from build123d import *

# Parameters (mm, degrees)
F1_DEPTH = 50.8
F3_DEPTH = 40.64
F0_R     = 12.7
F4_DEPTH = 50.8
F5_DEPTH = 38.1


with BuildPart() as f1:
    # F0 (on Front) → F1 (new body)
    with BuildSketch(Plane.XZ):
        with BuildLine():
            Line((-63.5, -50.8), (63.5, -50.8))
            ThreePointArc((63.5, -50.8), (72.480256, -47.080256), (76.2, -38.1))
            Line((76.2, -38.1), (76.2, 38.1))
            ThreePointArc((76.2, 38.1), (72.480256, 47.080256), (63.5, 50.8))
            Line((63.5, 50.8), (-63.5, 50.8))
            ThreePointArc((-63.5, 50.8), (-72.480256, 47.080256), (-76.2, 38.1))
            Line((-76.2, 38.1), (-76.2, -38.1))
            ThreePointArc((-76.2, -38.1), (-72.480256, -47.080256), (-63.5, -50.8))
        make_face()
    extrude(amount=-F1_DEPTH)

    # F2 (on face) → F3 (cut)
    with BuildSketch(Plane.XZ):
        with BuildLine():
            Line((-57.15, -44.45), (57.15, -44.45))
            ThreePointArc((57.15, -44.45), (66.130256, -40.730256), (69.85, -31.75))
            Line((69.85, -31.75), (69.85, 31.75))
            ThreePointArc((69.85, 31.75), (66.130256, 40.730256), (57.15, 44.45))
            Line((57.15, 44.45), (-57.15, 44.45))
            ThreePointArc((-57.15, 44.45), (-66.130256, 40.730256), (-69.85, 31.75))
            Line((-69.85, 31.75), (-69.85, -31.75))
            ThreePointArc((-69.85, -31.75), (-66.130256, -40.730256), (-57.15, -44.45))
        make_face()
    extrude(amount=-F3_DEPTH, mode=Mode.SUBTRACT)

    # F0 (on Front) → F4 (join)
    with BuildSketch(Plane.XZ):
        Polygon((-63.5, 50.8), (63.5, 50.8), (63.5, 76.2), (63.5, 101.6), (0, 101.6), (-38.1, 101.6), (-63.5, 101.6), align=None)
        with BuildLine():
            ThreePointArc((-25.4, 76.2), (-47.080256, 67.219744), (-38.1, 88.9))
            ThreePointArc((-38.1, 88.9), (-29.119744, 85.180256), (-25.4, 76.2))
        make_face(mode=Mode.SUBTRACT)
        with BuildLine():
            ThreePointArc((21.59, 76.2), (-15.266435, 60.933565), (0, 97.79))
            ThreePointArc((0, 97.79), (15.266435, 91.466435), (21.59, 76.2))
        make_face(mode=Mode.SUBTRACT)
        with Locations((38.1, 76.2)):
            Circle(F0_R, mode=Mode.SUBTRACT)
        with Locations((38.1, 76.2)):
            Circle(F0_R)
        with BuildLine():
            ThreePointArc((21.59, 76.2), (15.266435, 91.466435), (0, 97.79))
            ThreePointArc((0, 97.79), (-15.266435, 60.933565), (21.59, 76.2))
        make_face()
        with BuildLine():
            ThreePointArc((-25.4, 76.2), (-29.119744, 85.180256), (-38.1, 88.9))
            ThreePointArc((-38.1, 88.9), (-47.080256, 67.219744), (-25.4, 76.2))
        make_face()
    extrude(amount=-F4_DEPTH)

    # F0 (on Front) → F5 (cut)
    with BuildSketch(Plane.XZ):
        with BuildLine():
            ThreePointArc((-25.4, 76.2), (-29.119744, 85.180256), (-38.1, 88.9))
            ThreePointArc((-38.1, 88.9), (-47.080256, 67.219744), (-25.4, 76.2))
        make_face()
        with BuildLine():
            ThreePointArc((21.59, 76.2), (15.266435, 91.466435), (0, 97.79))
            ThreePointArc((0, 97.79), (-15.266435, 60.933565), (21.59, 76.2))
        make_face()
        with Locations((38.1, 76.2)):
            Circle(F0_R)
    extrude(amount=-F5_DEPTH, mode=Mode.SUBTRACT)


solid = f1.part
Input: part model. Units: mm. Frame: model coordinates. A direction names the side the tool comes from. Round coordinates to 2 decimals unless told otherwise and drop trailing zeros. Order: outer loops, then holes, each group sorted by start corner. A loop starts at its lowest first (then second) coordinate and runs counter-clockwise, first axis right, second up.
1. Set-up query: faces 4 (the face through (38, 38.1, 76)), 5 (the face through (-63.5, 25, 77)), 6 (the face through (1, 25, 101.6)). Return all of +Z, -Z, +X, -X, +Y, -Y with unobstructed straight access to the full face (end or side cutting, diameter ignored); none if empty.
The answers:
face 4: -Y
face 5: +Z, -X, +Y, -Y
face 6: +Z, +X, -X, +Y, -Y
2. Mould query, pull axis X, two halves, no side actions, for faces 1 (the face through (72.58, 25.04, 46.98)), 2 (the face through (1, 20, 44.45)), 3 (the face through (-1, 50.8, 26)). Classes: released by +X, released by -X, zero draft, split by the parting line, or undercut.
The answers:
face 1: released by +X
face 2: undercut
face 3: zero draft
3. Cut plane C-C, the plane x = 38.1. Output: boundary loops of the cut face in (y, z), then the cut area to 3 significant figures.
The answers:
outline: (0, -50.8) - (50.8, -50.8) - (50.8, 101.6) - (0, 101.6) - (0, 88.9) - (38.1, 88.9) - (38.1, 63.5) - (0, 63.5) - (0, 44.45) - (40.64, 44.45) - (40.64, -44.45) - (0, -44.45) - close
area: 3,160 mm2
4. Cut plane D-D, the plane x = -5.5. Output: boundary loops of the cut face in (y, z).
The answers:
outline: (0, -50.8) - (50.8, -50.8) - (50.8, 101.6) - (0, 101.6) - (0, 97.08) - (38.1, 97.08) - (38.1, 55.32) - (0, 55.32) - (0, 44.45) - (40.64, 44.45) - (40.64, -44.45) - (0, -44.45) - close
5. Material intervals for line 1 (Z direction, x = -38, y = 28); line 2 (X direction, y = 26.5, z = 27.5); line 3 (Z direction, x = 28.5, y = 23), sorted ascending.
The answers:
line 1: z = -50.8 to -44.45, 44.45 to 63.5, 88.9 to 101.6
line 2: x = -76.2 to -69.85, 69.85 to 76.2
line 3: z = -50.8 to -44.45, 44.45 to 67.89, 84.51 to 101.6
6. Cut plane A-A, the plane y = 20.5. Output: boundary loops of the cut face in (x, z).
The answers:
outline: (-76.2, -38.1) arc R12.7 ccw to (-63.5, -50.8) - (63.5, -50.8) arc R12.7 ccw to (76.2, -38.1) - (76.2, 38.1) arc R12.7 ccw to (63.5, 50.8) - (63.5, 101.6) - (-63.5, 101.6) - (-63.5, 50.8) arc R12.7 ccw to (-76.2, 38.1) - close; hole (-69.85, -31.75) arc R12.7 ccw to (-57.15, -44.45) - (57.15, -44.45) arc R12.7 ccw to (69.85, -31.75) - (69.85, 31.75) arc R12.7 ccw to (57.15, 44.45) - (-57.15, 44.45) arc R12.7 ccw to (-69.85, 31.75) - close; hole circle Ø25.4 at (-38.1, 76.2); hole (0, 97.79) arc R21.59 ccw (long way) to (21.59, 76.2) arc R21.59 ccw to start; hole circle Ø25.4 at (38.1, 76.2)
7. Cut plane B-B, the plane z = -28. Output: boundary loops of the cut face in (x, y).
The answers:
outline: (-76.2, 0) - (-69.85, 0) - (-69.85, 40.64) - (69.85, 40.64) - (69.85, 0) - (76.2, 0) - (76.2, 50.8) - (-76.2, 50.8) - close
8. Pin query (flat end, axial travel): P1, Ø6, axis at y = 18, z = 76, coming from the +X side; P2, Ø20.5, axis at x = -42, z = 71.5, coming from the -Y side; P3, Ø4, axis at y = 14, z = 46, coming from the +X side; P4, Ø10, axis at x = 42.5, z = 6.5, coming from the -Y side. Return the tip coordinate at first contact, or that it passes through.
The answers:
P1: stops at x = 63.5
P2: stops at y = 0
P3: stops at x = 74.75
P4: stops at y = 40.64
